Build history of the part. All positions in model axes, mm. Round coordinates to 2 decimals unless told otherwise and drop trailing zeros. Order: outer loops, then holes, each group sorted by start corner. A loop starts at its lowest first (then second) coordinate and runs counter-clockwise, first axis right, second up. Notation, with made-up numbers: M 46,79.25 L 99,79.25 A13 ccw 99,97.25 Z; hole C 25,-2 d6. An arc over 180 degrees is marked long. One line per question, with ' | ' between items. Start each with the question number.
Autodesk Inventor part; units mm, degrees
ref_plane "YZ Plane" through (0, 0, 0) normal (1, 0, 0) x (0, 1, 0)
ref_plane "XZ Plane" through (0, 0, 0) normal (0, 1, 0) x (-1, 0, 0)
ref_plane "XY Plane" through (0, 0, 0) normal (0, 0, 1) x (1, 0, 0)
sketch "Sketch1" plane through (0, 0, 0) normal (0, 0, 1) x (1, 0, 0)
  circle A0 centre (0, 0) radius 355
  dimension "d0" = 710
extrude "Plate1" add sketch "Sketch1" against normal blind 4
sketch "Sketch2" plane through (0, 0, 0) normal (0, 0, 1) x (1, 0, 0)
  circle A0 centre (0, 0) radius 320 construction
  circle A1 centre (0, 320) radius 16.5
  dimension "d2" = 640
  dimension "d3" = 33
extrude "Extrusion1" cut sketch "Sketch2" against normal through all
pattern_circular "Circular Pattern1" count 20 over 360 about axis through (0, 0, -10) along (0, 0, 1) of "Extrusion1"
equation "\"d1\" = Thickness"
equation "\"BendReliefWidth\" = Thickness"
equation "\"BendReliefDepth\" = 0.5 * Thickness"
equation "\"CornerReliefSize\" = 4 * Thickness"
equation "\"MinimumRemnant\" = 2 * Thickness"
equation "\"TransitionRadius\" = BendRadius"
equation "\"JacobiRadiusSize\" = BendRadius"
equation "\"GapSize\" = Thickness"
properties part number "MSC 037 flange cover 500" material "Stainless Steel"
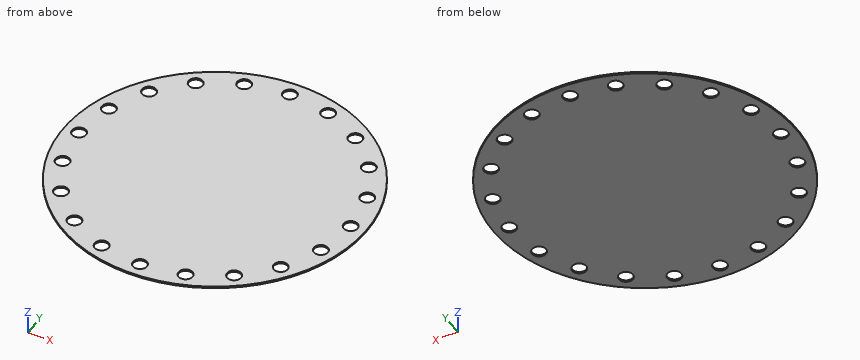
Item 1: Wall check: line 1 along Y through (x, z) = (84, -0.9); line 2 along Y through (x, z) = (-174, -3.3); line 3 along X through (y, z) = (202, -2.5). Give the ranges that are in metal, low to high. Write a range as [from, to].
Item 2: Flat gauge pins, fed straight in: pin 1 (1 mm diameter, centred on x = 194.5, z = -1, fed in from +Y); pin 2 (1 mm diameter, centred on y = 273.5, z = -3.5, fed in from -X); pin 3 (1 mm diameter, centred on x = 142, y = 77, fed in from +Z). Where does each tip first touch, or does it go through?
Item 3: Cut at D-D on x = -215.5. Write the cut outline in (y, z), then the cut area to 3 significant figures.
Item 4: Cut at A-A on y = 0. Write the cut outline in (x, z).
Item 5: Cut at C-C on z = -0.95. Count the separate pieces of the cut face and the enclosed holes in it, then the cut area to 3 significant figures.
Results found:
1) line 1: y = [-344.92, -311.46], [-297.22, 297.22], [311.46, 344.92] | line 2: y = [-309.43, -267.47], [-250.3, 250.3], [267.47, 309.43] | line 3: x = [-291.93, -267.76], [-250.01, 250.01], [267.76, 291.93]
2) pin 1: stops at y = 297.3 | pin 2: stops at x = -226.93 | pin 3: stops at z = 0
3) outline: M -282.11,-4 L 282.11,-4 L 282.11,0 L -282.11,0 Z | area: 2,260 mm^2
4) outline: M -355,-4 L -336.5,-4 L -336.5,0 L -355,0 Z; M -303.5,-4 L 303.5,-4 L 303.5,0 L -303.5,0 Z; M 336.5,-4 L 355,-4 L 355,0 L 336.5,0 Z
5) separate pieces: 1 | enclosed holes: 20 | area: 379,000 mm^2
